Model file for the job. Use its own axes, mm. Face numbers are marked on the shaded views. A direction names the side the tool comes from. Round coordinates to 2 decimals unless told otherwise and drop trailing zeros. Loops run counter-clockwise (first coordinate to the right, second up) from the corner with the lowest first, then second, coordinate; pieces in that order, holes last. Notation, with made-up numbers: M -33.5,-16 L 5.5,-16 A26 ccw 5.5,5 Z; hole C -7,14.25 d9. An arc over 180 degrees is marked long. Answer in a Markdown table with one row per item.
from build123d import *

# Parameters (mm, degrees)
F0_R     = 101.6
F1_DEPTH = 19.05
F2_R     = 15.875
F3_DEPTH = 12.7
F4_R     = 11.1125
F5_DEPTH = 19.05
F6_D     = 5.1054
F6_DEPTH = 19.05
F6_TIP   = 1.5338169022


with BuildPart() as f1:
    # F0 (on Front) → F1 (new body)
    with BuildSketch(Plane.XZ):
        with Locations((4.050075005, 0)):
            Circle(F0_R)
    extrude(amount=F1_DEPTH)

    # F2 (on face) → F3 (cut)
    with BuildSketch(Plane.XZ.offset(19.05)):
        with Locations((31.5849, 76.2762)):
            Circle(F2_R)
        with Locations((76.2762, 31.5849)):
            Circle(F2_R)
    extrude(amount=-F3_DEPTH, mode=Mode.SUBTRACT)

    # F4 (on face) → F5 (cut)
    with BuildSketch(Plane.XZ.offset(19.05)):
        Circle(F4_R)
    extrude(amount=-F5_DEPTH, mode=Mode.SUBTRACT)

    # F6
    with Locations(Plane.XZ.offset(19.05)):
        with Locations((36.449, 88.011), (26.7208, 64.5414), (88.011, 36.449), (64.5414, 26.7208)):
            Hole(F6_D / 2, depth=F6_DEPTH)
            with Locations((0, 0, -(F6_DEPTH + F6_TIP / 2))):  # 118° drill point
                Cone(0, F6_D / 2, F6_TIP, mode=Mode.SUBTRACT)


solid = f1.part
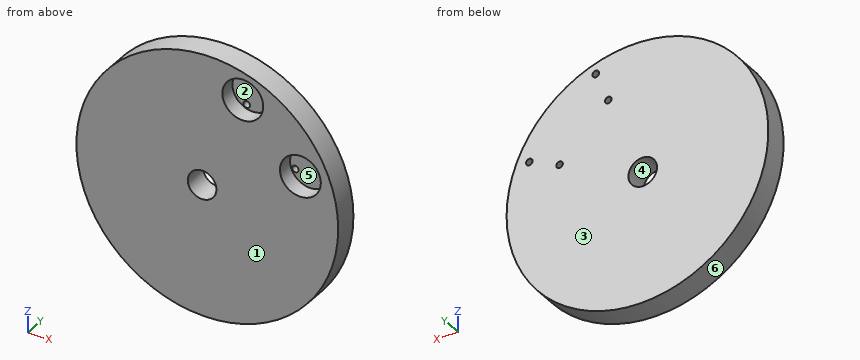
1. Wall check: probe 1 along X at (y, z) = (-15, 67); probe 2 along Z at (x, y) = (5.5, -12.25); probe 3 along X at (y, z) = (-14.75, -5.5). Give the ranges that are in metal, low to high.
Verdict:
| item | result |
|---|---|
| probe 1 | x = -72.33 to 18.7, 44.47 to 80.43 |
| probe 2 | z = -101.59 to -9.66, 9.66 to 101.59 |
| probe 3 | x = -97.4 to -9.66, 9.66 to 105.5 |
2. Saw through at D-D (x = 58). Write the cut outline in (y, z).
Verdict:
| item | result |
|---|---|
| outline | M -19.05,-86.09 L 0,-86.09 L 0,86.09 L -19.05,86.09 Z |
3. Saw through at B-B (x = 0). Write the cut outline in (y, z).
Verdict:
| item | result |
|---|---|
| outline | M -19.05,-101.52 L 0,-101.52 L 0,-11.11 L -19.05,-11.11 Z; M -19.05,11.11 L 0,11.11 L 0,101.52 L -19.05,101.52 Z |
4. Mould opens along Z. For the marked faces 3, 4, 5 and 6 say: +Z half, -Z half, draft (parallel to the pull), parting line (faces both ways), or undercut.
Verdict:
| item | result |
|---|---|
| face 3 | draft |
| face 4 | undercut |
| face 5 | undercut |
| face 6 | parting line |
5. Saw through at C-C (y = -11). State how many separate pieces and enclosed holes the cut face has, and give its area (3 significant figures).
Verdict:
| item | result |
|---|---|
| separate pieces | 1 |
| enclosed holes | 3 |
| area | 30,500 mm² |
6. Pin check, flat tips, straight feed: pin 1 (10 mm diameter, centred on x = -73.5, y = -5.5, fed in from +Z); pin 2 (4 mm diameter, centred on x = 26.72, z = 64.54, fed in from -Y); pin 3 (5 mm diameter, centred on y = -7, z = -1.5, fed in from -X); pin 4 (6 mm diameter, centred on x = 64.54, z = 26.72, fed in from -Y). Stop position of each tip, or through.
Verdict:
| item | result |
|---|---|
| pin 1 | stops at z = 71.13 |
| pin 2 | passes through |
| pin 3 | stops at x = -97.55 |
| pin 4 | stops at y = -6.35 |
7. Tool access for the marked faces 1 and 2: list every direction of +Z, -Z, +X, -X, +Y, -Y with a clear straight run to the whole face (end or side of a thin tool).
Verdict:
| item | result |
|---|---|
| face 1 | +Z, -Z, +X, -X, -Y |
| face 2 | -Y |
8. Saw through at A-A (z = 0). Write the cut outline in (x, y), and give its area (3 significant figures).
Verdict:
| item | result |
|---|---|
| outline | M -97.55,-19.05 L -11.11,-19.05 L -11.11,0 L -97.55,0 Z; M 11.11,-19.05 L 105.65,-19.05 L 105.65,0 L 11.11,0 Z |
| area | 3,450 mm² |
